CAD build for the part. Positions are in the model's coordinates, mm. Round coordinates to 2 decimals unless told otherwise and drop trailing zeros. Write each loop counter-clockwise with the first axis right and the second up, starting at its lowest first coordinate (ties: lowest second). Pieces come first, ordered by that corner, then holes. Notation, with made-up numbers: (32, 17.25) - (59, 17.25) arc R9 cw to (59, 30.25) - close; hole circle Ø8 at (80.5, -4). An arc over 180 degrees is marked (long way). Put each result on its own line as item: value. Start each with the question number.
Item 1: Mould opens along Z. For faces 1 (the cylindrical face through (-25.35, -23.466, 83.175)), 2 (the flat face through (-25, -25, 150)), 3 (the flat face through (-25, 0, 73)) say: released by +Z, released by -Z, zero draft, split by the parting line, or undercut.
Item 2: Cut at A-A (y = -19.5). Give the cut face in (x, z), and give its area (3 significant figures).
Item 3: Cut at C-C (y = -35). Give the cut face in (x, z).
Item 4: Cut at B-B (x = -9). Give the cut face in (y, z).
Item 5: Pin check, flat tips, straight feed: pin 1 Ø5 at (y, z) = (-19, 81.5) entering from +X; pin 2 Ø14 at (y, z) = (-25, 71.49) entering from +X. Stop position of each tip, or through.
Item 6: Drill centre lines: line 1 (Z direction, x = -22, y = -25); line 2 (Z direction, x = -19.5, y = -27); line 3 (Y direction, x = -41, z = 78). Where is each one in solid material? Low to high. Write a range as from..to.
```python
from build123d import *

# Parameters (mm, degrees)
F0_W     = 50
F0_H     = 50
F1_DEPTH = 150
F2_R     = 11.784689
F3_DEPTH = 131.62777
F4_SIZE  = 2


with BuildPart() as f1:
    # F0 (on Top) → F1 (new body)
    with BuildSketch(Plane.XY):
        with Locations((-25, -25)):
            Rectangle(F0_W, F0_H)
    extrude(amount=F1_DEPTH)

    # F2 (on face) → F3 (cut)
    with BuildSketch(Plane(origin=(-50, 0, 0), x_dir=(0, -1, 0), z_dir=(-1, 0, 0))):
        with Locations((25, 71.490675)):
            Circle(F2_R)
    extrude(amount=-F3_DEPTH, mode=Mode.SUBTRACT)

    # F4
    f4_edges = [f1.edges().sort_by_distance(p)[0] for p in [
        (-50, -25, 150),
        (0, -25, 150),
        (-25, -50, 150),
        (-25, 0, 150),
    ]]
    chamfer(f4_edges, length=F4_SIZE)


solid = f1.part
```
Output values:
1. face 1: undercut
1. face 2: released by +Z
1. face 3: zero draft
2. outline: (-50, 0) - (0, 0) - (0, 61.07) - (-50, 61.07) - close; (-50, 81.91) - (0, 81.91) - (0, 148) - (-2, 150) - (-48, 150) - (-50, 148) - close
2. area: 6,450 mm2
3. outline: (-50, 0) - (0, 0) - (0, 65.26) - (-50, 65.26) - close; (-50, 77.73) - (0, 77.73) - (0, 148) - (-2, 150) - (-48, 150) - (-50, 148) - close
4. outline: (-50, 0) - (0, 0) - (0, 148) - (-2, 150) - (-48, 150) - (-50, 148) - close; hole circle Ø23.57 at (-25, 71.49)
5. pin 1: x = 0
5. pin 2: through
6. line 1: 0..59.71, 83.28..150
6. line 2: 0..59.88, 83.1..150
6. line 3: -50..-34.82, -15.18..0
